Input: dimensioned drawing with shaded views. Units: mm. Origin: part minimum x, y, z. Round coordinates to 2 decimals unless told otherwise and drop trailing zeros. Loops run counter-clockwise (first coordinate to the right, second up) from the corner with the lowest first, then second, coordinate; pieces in that order, holes last.
1) Section A-A, the plane z = 1.25. Return loops of the section in (x, y), and give its area (3 significant figures).
2) First-contact query: pin 1 (2 mm diameter, centred on x = 5.08, y = 5.08, fed in from -Z) (1 decimal). Flat tip, straight axial feed; report the tip coordinate or a pass-through.
3) Section B-B, the plane y = 9. Return loops of the section in (x, z).
4) Ray query, line 1 along Y through (x, z) = (5.08, 1.5); line 2 along X through (y, z) = (5.75, 2); line 3 along X through (y, z) = (4.75, 1). Return the intervals inside material, ascending.
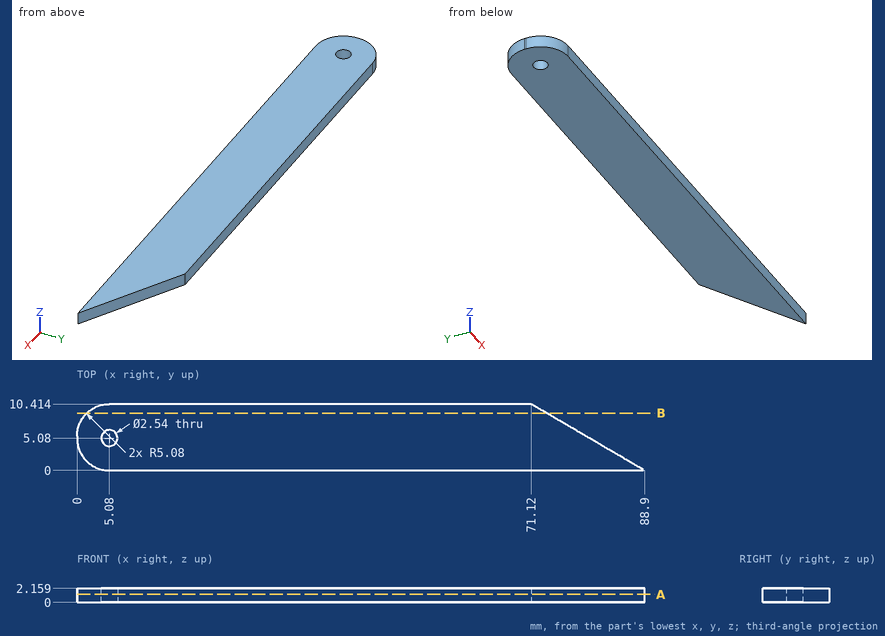
Final values:
1. outline: (0, 5.08) arc R5.08 ccw to (5.08, 0) - (88.9, 0) - (71.12, 10.41) - (5.08, 10.41) arc R5.08 ccw to (0, 5.33) - close; hole circle Ø2.54 at (5.08, 5.08)
1. area: 817 mm2
2. pin 1: passes through
3. outline: (1.56, 0) - (73.53, 0) - (73.53, 2.16) - (1.56, 2.16) - close
4. line 1: y = 0 to 3.81, 6.35 to 10.41
4. line 2: x = 0.02 to 4, 6.16 to 79.08
4. line 3: x = 0.01 to 3.85, 6.31 to 80.79
